Input: part model. Units: mm. Frame: model coordinates. A direction names the side the tool comes from. Coordinates: 2 decimals unless noted, no trailing zeros. Loops run counter-clockwise (first coordinate to the right, second up) from the corner with the lowest first, then second, coordinate; pieces in that order, holes last.
Autodesk Inventor part; units mm, degrees
ref_plane "YZ Plane" through (0, 0, 0) normal (1, 0, 0) x (0, 1, 0)
ref_plane "XZ Plane" through (0, 0, 0) normal (0, 1, 0) x (-1, 0, 0)
ref_plane "XY Plane" through (0, 0, 0) normal (0, 0, 1) x (1, 0, 0)
sketch "スケッチ1" plane through (0, 0, 0) normal (0, 0, 1) x (1, 0, 0)
  line L0 (-12.5, 25) -> (12.5, 25)
  line L1 (12.5, 25) -> (12.5, -25)
  line L2 (12.5, -25) -> (-12.5, -25)
  line L3 (-12.5, -25) -> (-12.5, 25)
  line L4 (-10.5, 23) -> (10.5, 23)
  line L5 (10.5, 23) -> (10.5, -23)
  line L6 (10.5, -23) -> (-10.5, -23)
  line L7 (-10.5, -23) -> (-10.5, 23)
  point P0 (0, 0)
  dimension "d0" = 25
  dimension "d1" = 50
  dimension "d2" = 46
  dimension "d3" = 21
  dimension "d4" = 25
  dimension "d5" = 23
  dimension "d6" = 10.5
  dimension "d7" = 12.5
extrude "押し出し1" add sketch "スケッチ1" along normal blind 50
sketch "スケッチ2" plane through (-12.5, 25, 0) normal (0, 1, 0) x (1, 0, 0)
  line L0 (0, 0) -> (25, 0)
  line L1 (0, 0) -> (0, -50)
  arc A0 (6, -33.5) -> (19, -33.5) centre (12.5, -33.5) ccw
  line L2 (6, -33.5) -> (6, 0)
  line L3 (19, -33.5) -> (19, 0)
  point P0 (12.5, 0)
  dimension "d10" = 13
  dimension "d11" = 33.5
  dimension "d12" = 12.5
extrude "押し出し2" cut sketch "スケッチ2" against normal blind 2
sketch "スケッチ3" plane through (-12.5, 25, 50) normal (0, 1, 0) x (1, 0, 0)
  arc A0 (6, 16.5) -> (19, 16.5) centre (12.5, 16.5) ccw
  circle A1 centre (4.5, 10) radius 1
  circle A2 centre (4.5, 46) radius 1
  circle A3 centre (20.5, 46) radius 1
  circle A4 centre (20.5, 10) radius 1
  line L0 (19, 50) -> (25, 50)
  point P0 (12.5, 50)
  dimension "d15" = 6.5
  dimension "d16" = 6.5
  dimension "d17" = 2
  dimension "d18" = 8
  dimension "d19" = 8
  dimension "d20" = 8
  dimension "d21" = 8
  dimension "d22" = 29.5
  dimension "d23" = 29.5
  dimension "d119" = 4
hole "穴1" at (-8, 25, 4) at (8, 25, 4) at (8, 25, 40) at (-8, 25, 40) direction (0, -1, 0) diameter 2 depth 2 tip angle 118 counterbore diameter 4 counterbore depth 0.5
sketch "スケッチ4" plane through (-12.5, -25, 0) normal (0, -1, 0) x (1, 0, 0)
  line L0 (25, 0) -> (0, 0)
  line L1 (25, 0) -> (25, 50)
  circle A0 centre (12.5, 10.5) radius 2
  point P0 (12.5, 0)
  dimension "d31" = 4
  dimension "d32" = 12.5
  dimension "d33" = 10.5
hole "穴2" at (0, -25, 10.5) direction (0, 1, 0) diameter 4 end through all
sketch "スケッチ5" plane through (-12.5, 25, 50) normal (0, 1, 0) x (1, 0, 0)
  arc A0 (6, 16.5) -> (19, 16.5) centre (12.5, 16.5) ccw
  circle A1 centre (20.5, 4) radius 1.5
  circle A2 centre (4.5, 4) radius 1.5
  circle A3 centre (20.5, 10) radius 2
  circle A4 centre (4.5, 10) radius 2
  point P0 (12.5, 50)
  dimension "d46" = 8
  dimension "d47" = 8
  dimension "d57" = 3
  dimension "d120" = 6
  dimension "d121" = 6
hole "穴4" at (-8, 25, 46) at (8, 25, 46) direction (0, -1, 0) diameter 3 end through all
thread "ねじ1"
thread "ねじ2"
thread "ねじ3"
thread "ねじ4"
sketch "スケッチ7" plane through (-12.5, -25, 0) normal (0, -1, 0) x (1, 0, 0)
  line L0 (25, 0) -> (25, 50)
  circle A0 centre (12.5, 30) radius 4
  circle A1 centre (12.5, 10.5) radius 2
  point P0 (12.5, 0)
  dimension "d79" = 8
  dimension "d80" = 12.5
  dimension "d118" = 19.5
hole "穴5" at (0, -25, 30) direction (0, 1, 0) diameter 8 end through all
sketch "スケッチ8" plane through (12.5, -25, 0) normal (1, 0, 0) x (0, 0, -1)
  line L0 (-50, 50) -> (-50, 0)
  circle A0 centre (-27.5, 37.5) radius 1.5
  circle A1 centre (-27.5, 12.5) radius 1.5
  circle A2 centre (-7.5, 42.5) radius 1.5
  circle A3 centre (-7.5, 7.5) radius 1.5
  line L1 (0, 50) -> (0, 0)
  line L2 (0, 50) -> (-50, 50)
  point P0 (0, 25)
  dimension "d88" = 25
  dimension "d90" = 3
  dimension "d101" = 35
  dimension "d104" = 20
  dimension "d105" = 20
  dimension "d113" = 50
  dimension "d114" = 7.5
  dimension "d115" = 7.5
  dimension "d116" = 7.5
  dimension "d117" = 5
hole "穴7" at (12.5, 12.5, 27.5) at (12.5, -12.5, 27.5) at (12.5, -17.5, 7.5) at (12.5, 17.5, 7.5) direction (-1, 0, 0) diameter 3 end through all
properties part number "07" material "アルミニウム 6061"
Item 1: Contact query for flat-ended pins moving along their axis: P1, Ø2.5, axis at y = 17.5, z = 7.5, coming from the +X side; P2, Ø2.5, axis at x = -8, z = 4, coming from the +Y side. Output: stop coordinate, or through.
Result:
P1: passes through
P2: stops at y = 24.5
Item 2: Section query C-C (x = -8). Count the separate pieces of the cut face and the enclosed holes in it, then the cut area to 3 significant figures.
Result:
separate pieces: 6
enclosed holes: 0
area: 178 mm2
Item 3: Reachability of faces 1 (the face through (-10, 24.75, 4.07)), 2 (the face through (-8.07, 23.99, 44.5)), 3 (the face through (-10.5, 0, 25)) from +Z, -Z, +X, -X, +Y, -Y: full face, straight path, thin tool, end or side. Return the list, or none.
Result:
face 1: +Y
face 2: +Y, -Y
face 3: +Z, -Z
Item 4: Section query D-D (y = -5.5). Output: boundary loops of the cut face in (x, z).
Result:
outline: (-12.5, 0) - (-10.5, 0) - (-10.5, 50) - (-12.5, 50) - close; (10.5, 0) - (12.5, 0) - (12.5, 50) - (10.5, 50) - close
Item 5: Section query A-A (z = 4). Output: boundary loops of the cut face in (x, y), then the cut area to 4 significant figures.
Result:
outline: (-12.5, -25) - (12.5, -25) - (12.5, 25) - (10, 25) - (10, 24.5) - (9, 24.5) - (9, 23) - (10.5, 23) - (10.5, -23) - (-10.5, -23) - (-10.5, 23) - (-9, 23) - (-9, 24.5) - (-10, 24.5) - (-10, 25) - (-12.5, 25) - close; (-7, 23) - (-6.5, 23) - (-6.5, 24.5) - (-7, 24.5) - close; (6.5, 23) - (7, 23) - (7, 24.5) - (6.5, 24.5) - close
area: 248.5 mm2
Item 6: Line query: L1, parallel to Z at x = -8, y = 24.85; L2, parallel to X at y = 24, z = 4; L3, parallel to Z at x = 8, y = 23.9. Output: solid intervals per line, ascending.
Result:
L1: z = 0 to 2, 6 to 38, 42 to 44.5, 47.5 to 50
L2: x = -12.5 to -9, -7 to -6.5, 6.5 to 7, 9 to 12.5
L3: z = 0 to 3, 5 to 39, 41 to 44.5, 47.5 to 50
Item 7: Section query B-B (y = 12.5). Output: boundary loops of the cut face in (x, z), then the cut area to 3 significant figures.
Result:
outline: (-12.5, 0) - (-10.5, 0) - (-10.5, 26) - (-12.5, 26) - close; (-12.5, 29) - (-10.5, 29) - (-10.5, 50) - (-12.5, 50) - close; (10.5, 0) - (12.5, 0) - (12.5, 26) - (10.5, 26) - close; (10.5, 29) - (12.5, 29) - (12.5, 50) - (10.5, 50) - close
area: 188 mm2
Item 8: Mould query, pull axis Z, two halves, no side actions, for faces 4 (the face through (6.5, 24, 17)), 5 (the face through (0, 24, 40)), 6 (the face through (-11.51, 12.43, 29)). Classes: +Z half, -Z half, draft (parallel to the pull), parting line (faces both ways), or undercut.
Result:
face 4: draft
face 5: -Z half
face 6: undercut
